Part model, mm, in its own coordinate system. Coordinates: 2 decimals unless noted, no trailing zeros. Loops run counter-clockwise (first coordinate to the right, second up) from the corner with the lowest first, then second, coordinate; pieces in that order, holes last. Notation, with made-up numbers: (71, 9.25) - (114, 9.25) arc R21 cw to (114, 20.25) - close; hole circle Ø3 at (-12.75, -38.75). An arc over 180 degrees is marked (long way). Use a Markdown table: item, result. Add a question column.
1. Band-saw the part on C-C, the plane z = -82. Give the cut face in (x, y), plus the area to 3 significant figures.
2. Band-saw the part on A-A, the plane x = 0. Give the cut face in (y, z), plus the area to 3 significant figures.
3. Wall check: probe 1 along Y at (x, z) = (0, -37); probe 2 along X at (y, z) = (-10, -13); probe 3 along Y at (x, z) = (-1.5, 31). Give the ranges that are in metal, low to high. Write a range as [from, to].
4. Band-saw the part on B-B, the plane y = 10. Give the cut face in (x, z), plus the area to 3 significant figures.
from build123d import *

# Parameters (mm, degrees)
IZIM1_W                     = 17.5
IZIM1_H                     = 35
Y_KSEKLIK_EKSTR_ZYON1_DEPTH = 98
M5_DI_LI_DELIK1_AT_2_COUNT  = 2
M5_DI_LI_DELIK1_AT_2_PITCH  = 20


with BuildPart() as part:
    # Çizim1 → Yükseklik-Ekstrüzyon1 (new, symmetric)
    with BuildSketch(Plane.XY):
        Rectangle(IZIM1_W, IZIM1_H)
    extrude(amount=Y_KSEKLIK_EKSTR_ZYON1_DEPTH, both=True)

    # Çizim3 → M5 Dişli Delik1 (revolve, cut)
    with BuildSketch(Plane(origin=(0, 10, 98), x_dir=(0, -1, 0), z_dir=(1, 0, 0))):
        Polygon((0, 0), (0, 201.2618073), (2.1, 200), (2.1, 0), align=None)
    m5_di_li_delik1 = revolve(axis=Axis((0, 10, 104.35), (0, 0, -1)), mode=Mode.SUBTRACT)

    # M5 Dişli Delik1 at 2: M5 Dişli Delik1 ×2
    with Locations(*[(0, -i * M5_DI_LI_DELIK1_AT_2_PITCH, 0) for i in range(1, M5_DI_LI_DELIK1_AT_2_COUNT)]):
        add(m5_di_li_delik1, mode=Mode.SUBTRACT)

    # Aynalama1: M5 Dişli Delik1 across plane
    add(m5_di_li_delik1.mirror(Plane.XY), mode=Mode.SUBTRACT)

    # Aynalama1 copy 1 sketch → Aynalama1 copy 1 (revolve, cut)
    with BuildSketch(Plane(origin=(0, -10, -98), x_dir=(0, -1, 0), z_dir=(1, 0, 0))):
        Polygon((0, 0), (0, -201.2618073), (2.1, -200), (2.1, 0), align=None)
    revolve(axis=Axis((0, -10, -104.35), (0, 0, -1)), mode=Mode.SUBTRACT)


solid = part.part
Geometry check:
| question | item | result |
|---|---|---|
| 1 | outline | (-8.75, -17.5) - (8.75, -17.5) - (8.75, 17.5) - (-8.75, 17.5) - close; hole circle Ø4.2 at (0, -10); hole circle Ø4.2 at (0, 10) |
| 1 | area | 585 mm^2 |
| 2 | outline | (-17.5, -98) - (-12.1, -98) - (-12.1, 98) - (-17.5, 98) - close; (-7.9, -98) - (7.9, -98) - (7.9, 98) - (-7.9, 98) - close; (12.1, -98) - (17.5, -98) - (17.5, 98) - (12.1, 98) - close |
| 2 | area | 5,210 mm^2 |
| 3 | probe 1 | y = [-17.5, -12.1], [-7.9, 7.9], [12.1, 17.5] |
| 3 | probe 2 | x = [-8.75, -2.1], [2.1, 8.75] |
| 3 | probe 3 | y = [-17.5, -11.47], [-8.53, 8.53], [11.47, 17.5] |
| 4 | outline | (-8.75, -98) - (-2.1, -98) - (-2.1, 98) - (-8.75, 98) - close; (2.1, -98) - (8.75, -98) - (8.75, 98) - (2.1, 98) - close |
| 4 | area | 2,610 mm^2 |
